Geometry check sheet. Reference: the model listing, model coordinates, mm. A direction names the side the tool comes from. Round coordinates to 2 decimals unless told otherwise and drop trailing zeros. Loops run counter-clockwise (first coordinate to the right, second up) from the corner with the lowest first, then second, coordinate; pieces in that order, holes last. Notation, with made-up numbers: (74.5, 55.25) - (123.5, 55.25) arc R26 ccw to (123.5, 72.25) - close; hole circle Ø2 at (16.25, -24.5). An arc over 180 degrees is marked (long way). Write item = value, one per line.
```python
from build123d import *

# Parameters (mm, degrees)
SKETCH_1_R               = 3.5
EXTRUDE_1_DEPTH          = 3
SKETCH_2_R               = 3
SKETCH_2_R_2             = 2.1
CUT_EXTRUDE_1_DEPTH      = 10
SKETCH_4_R               = 2.1
CUT_EXTRUDE_3_DEPTH      = 10
CHAMFER_1_SIZE           = 10
FILLET_1_R               = 3
SKETCH_5_R               = 2.1
CUT_EXTRUDE_4_DEPTH      = 10
SKETCH_3_R               = 1.6
CUT_EXTRUDE_5_DEPTH      = 10
EXTRUDE_2_DEPTH          = 6
CUT_EXTRUDE_6_DEPTH      = 182.747077005
CUT_EXTRUDE_6_DEPTH_BACK = 182.747077005
SKETCH_6_3_R             = 6.025
FILLET_2_R               = 6
SKETCH_7_R               = 2.1
EXTRUDE_3_DEPTH          = 6
FILLET_3_R               = 3


with BuildPart() as part:
    # 草图1 → 凸台-拉伸1 (new, symmetric)
    with BuildSketch(Plane(origin=(0, 0, 0), x_dir=(0, 0, -1), z_dir=(1, 0, 0))):
        with BuildLine():
            Line((-60, -42.021540511), (0, -70))
            Line((0, -70), (12, -70))
            Line((12, -70), (12, 30))
            Line((12, 30), (-75.715728753, 30))
            Line((-75.715728753, 30), (-125.857864376, 80.142135624))
            ThreePointArc((-125.857864376, 80.142135624), (-154.142135624, 80.142135624), (-154.142135624, 51.857864376))
            Line((-154.142135624, 51.857864376), (-92.284271247, -10))
            Line((-92.284271247, -10), (-60, -10))
            Line((-60, -10), (-60, -42.021540511))
        make_face()
        Circle(SKETCH_1_R, mode=Mode.SUBTRACT)
    extrude(amount=EXTRUDE_1_DEPTH, both=True)

    # 草图2 → 切除-拉伸1 (cut)
    with BuildSketch(Plane(origin=(3, 0, 0), x_dir=(0, 0, -1), z_dir=(1, 0, 0))):
        with Locations((-140, 66)):
            Circle(SKETCH_2_R)
        with Locations((-140, 82)):
            Circle(SKETCH_2_R_2)
        with Locations((-126.143593539, 74)):
            Circle(SKETCH_2_R_2)
        with Locations((-126.143593539, 58)):
            Circle(SKETCH_2_R_2)
        with Locations((-140, 50)):
            Circle(SKETCH_2_R_2)
        with Locations((-153.856406461, 58)):
            Circle(SKETCH_2_R_2)
        with Locations((-153.856406461, 74)):
            Circle(SKETCH_2_R_2)
    extrude(amount=-CUT_EXTRUDE_1_DEPTH, mode=Mode.SUBTRACT)

    # 草图4 → 切除-拉伸3 (cut)
    with BuildSketch(Plane(origin=(3, 0, 0), x_dir=(0, 0, -1), z_dir=(1, 0, 0))):
        with Locations((-55, -15)):
            Circle(SKETCH_4_R)
        with Locations((-55, -35)):
            Circle(SKETCH_4_R)
        with Locations((7, -65)):
            Circle(SKETCH_4_R)
        with Locations((7, -45)):
            Circle(SKETCH_4_R)
        with Locations((-8, -60.75264914)):
            Circle(SKETCH_4_R)
        with Locations((-26.126155741, -52.300283905)):
            Circle(SKETCH_4_R)
        with Locations((-44.252311481, -43.84791867)):
            Circle(SKETCH_4_R)
    extrude(amount=-CUT_EXTRUDE_3_DEPTH, mode=Mode.SUBTRACT)

    # 倒角1
    chamfer_1_edges = [part.edges().sort_by_distance(p)[0] for p in [
        (0, -10, 60),
    ]]
    chamfer(chamfer_1_edges, length=CHAMFER_1_SIZE)

    # 圆角1
    fillet_1_edges = [part.edges().sort_by_distance(p)[0] for p in [
        (0, -20, 60),
        (0, -10, 70),
        (0, 30, -12),
        (0, -70, -12),
        (0, -70, 0),
        (0, -42.021540511, 60),
        (0, -10, 92.284271247),
        (0, 30, 75.715728753),
    ]]
    fillet(fillet_1_edges, radius=FILLET_1_R)

    # 草图5 → 切除-拉伸4 (cut)
    with BuildSketch(Plane(origin=(3, 0, 0), x_dir=(0, 0, -1), z_dir=(1, 0, 0))):
        with Locations((-110, 57.213203436)):
            Circle(SKETCH_5_R)
        with Locations((-88.786796564, 36)):
            Circle(SKETCH_5_R)
        with Locations((-109.946763354, 14.785654888)):
            Circle(SKETCH_5_R)
        with Locations((-131.214342006, 35.94434337)):
            Circle(SKETCH_5_R)
        with Locations((-58, 25)):
            Circle(SKETCH_5_R)
        with Locations((-28, 25)):
            Circle(SKETCH_5_R)
    extrude(amount=-CUT_EXTRUDE_4_DEPTH, mode=Mode.SUBTRACT)

    # 草图3 → 切除-拉伸5 (cut)
    with BuildSketch(Plane(origin=(3, 0, 0), x_dir=(0, 0, -1), z_dir=(1, 0, 0))):
        with Locations((0, 8)):
            Circle(SKETCH_3_R)
        with Locations((6.92820323, 4)):
            Circle(SKETCH_3_R)
        with Locations((6.92820323, -4)):
            Circle(SKETCH_3_R)
        with Locations((0, -8)):
            Circle(SKETCH_3_R)
        with Locations((-6.92820323, -4)):
            Circle(SKETCH_3_R)
        with Locations((-6.92820323, 4)):
            Circle(SKETCH_3_R)
    extrude(amount=-CUT_EXTRUDE_5_DEPTH, mode=Mode.SUBTRACT)

    # 草图6 → 凸台-拉伸2 (add)
    with BuildSketch(Plane(origin=(3, 0, 0), x_dir=(0, 0, -1), z_dir=(1, 0, 0))):
        with BuildLine():
            ThreePointArc((-51.06307787, -50.273817383), (-46.226182617, -63.56307787), (-32.93692213, -58.726182617))
            ThreePointArc((-32.93692213, -58.726182617), (-32.302787653, -56.942145102), (-32.016290131, -55.070558726))
            Line((-32.016290131, -55.070558726), (-36.127383127, -53.153524579))
            ThreePointArc((-36.127383127, -53.153524579), (-36.013216988, -53.822464636), (-35.975, -54.5))
            ThreePointArc((-35.975, -54.5), (-45.144179406, -59.639529245), (-44.743385348, -49.13581676))
            Line((-44.743385348, -49.13581676), (-48.854478344, -47.218782613))
            ThreePointArc((-48.854478344, -47.218782613), (-50.10403963, -48.64128498), (-51.06307787, -50.273817383))
        make_face()
        with BuildLine():
            Line((-49.498462108, -46.918488052), (-51.06307787, -50.273817383))
            ThreePointArc((-51.06307787, -50.273817383), (-50.10403963, -48.64128498), (-48.854478344, -47.218782613))
            Line((-48.854478344, -47.218782613), (-49.498462108, -46.918488052))
        make_face()
        with BuildLine():
            ThreePointArc((-32.016290131, -55.070558726), (-32.302787653, -56.942145102), (-32.93692213, -58.726182617))
            Line((-32.93692213, -58.726182617), (-31.372306367, -55.370853287))
            Line((-31.372306367, -55.370853287), (-32.016290131, -55.070558726))
        make_face()
    extrude(amount=-EXTRUDE_2_DEPTH)

    # 草图6<3> → 切除-拉伸6 (cut, two sides: drawn at the far end of the back side and taken through both)
    with BuildSketch(Plane(origin=(3, 0, 0), x_dir=(0, 0, -1), z_dir=(1, 0, 0)).offset(-CUT_EXTRUDE_6_DEPTH_BACK)):
        with Locations((-42, -54.5)):
            Circle(SKETCH_6_3_R)
    extrude(amount=CUT_EXTRUDE_6_DEPTH + CUT_EXTRUDE_6_DEPTH_BACK, mode=Mode.SUBTRACT)

    # 圆角2
    fillet_2_edges = [part.edges().sort_by_distance(p)[0] for p in [
        (0, -46.918488052, 49.498462108),
        (0, -55.370853287, 31.372306367),
    ]]
    fillet(fillet_2_edges, radius=FILLET_2_R)

    # 草图7 → 凸台-拉伸3 (add)
    # profile 1 of 2: a face of its own
    with BuildSketch(Plane(origin=(3, 0, 0), x_dir=(0, 0, -1), z_dir=(1, 0, 0))):
        with BuildLine():
            Line((-61.377870017, 57.235829935), (-132.83107829, 84.671008583))
            ThreePointArc((-132.83107829, 84.671008583), (-129.106517373, 82.772955502), (-125.857864376, 80.142135624))
            Line((-125.857864376, 80.142135624), (-111.475100576, 65.759371824))
            Line((-111.475100576, 65.759371824), (-64.962330872, 47.900325644))
            Line((-64.962330872, 47.900325644), (-63.922837224, 50.607621888))
            ThreePointArc((-63.922837224, 50.607621888), (-65.130556346, 53.320814569), (-62.417363665, 54.528533691))
            Line((-62.417363665, 54.528533691), (-61.377870017, 57.235829935))
        make_face()
        with Locations((-81.841109028, 59.736999499)):
            Circle(SKETCH_7_R, mode=Mode.SUBTRACT)
    # profile 2 of 2: a face of its own
    with BuildSketch(Plane(origin=(3, 0, 0), x_dir=(0, 0, -1), z_dir=(1, 0, 0))):
        with BuildLine():
            Line((10.075338256, 29.800651288), (-61.377870017, 57.235829935))
            Line((-61.377870017, 57.235829935), (-62.417363665, 54.528533691))
            ThreePointArc((-62.417363665, 54.528533691), (-61.439385673, 53.757458461), (-61.070100444, 52.56807779))
            ThreePointArc((-61.070100444, 52.56807779), (-61.980719773, 50.837363019), (-63.922837224, 50.607621888))
            Line((-63.922837224, 50.607621888), (-64.962330872, 47.900325644))
            Line((-64.962330872, 47.900325644), (-18.342051383, 30))
            Line((-18.342051383, 30), (9, 30))
            ThreePointArc((9, 30), (9.546830018, 29.949741841), (10.075338256, 29.800651288))
        make_face()
        with Locations((-44.499091861, 45.39915608)):
            Circle(SKETCH_7_R, mode=Mode.SUBTRACT)
    extrude(amount=-EXTRUDE_3_DEPTH)

    # 圆角3
    fillet_3_edges = [part.edges().sort_by_distance(p)[0] for p in [
        (0, 65.759371824, 111.475100576),
        (0, 30, 18.342051383),
    ]]
    fillet(fillet_3_edges, radius=FILLET_3_R)


solid = part.part
```
(1) Gauge pin test, flat ends, axial feed: pin 1 (2.5 mm diameter, centred on y = 4, z = 6.93, fed in from +X); pin 2 (2 mm diameter, centred on x = -1.5, y = -16, fed in from +Z); pin 3 (3 mm diameter, centred on x = 1, z = 42.5, fed in from +Y); pin 4 (1 mm diameter, centred on x = 0.5, y = -5.5, fed in from +Z). Record the tip position at first contact, or that the pin passes through.
Answers follow:
pin_1 = through
pin_2 = 65
pin_3 = 50.56
pin_4 = 97.28
(2) Section check A-A (y = -35). Enter the section's corners in (x, z), then the cut area to 3 significant figures.
Answers follow:
outline = (-3, -12) - (3, -12) - (3, 52.9) - (-3, 52.9) - close; (-3, 57.1) - (3, 57.1) - (3, 60) - (-3, 60) - close
area = 407 mm²
(3) Section check C-C (x = -0.5). State how many separate pieces and enclosed holes the cut face has, then the cut area to 3 significant figures.
Answers follow:
separate_pieces = 1
enclosed_holes = 32
area = 12,200 mm²
(4) Section check B-B (y = 25). Enter the section's corners in (x, z).
Answers follow:
outline = (-3, -12) - (3, -12) - (3, 25.9) - (-3, 25.9) - close; (-3, 30.1) - (3, 30.1) - (3, 55.9) - (-3, 55.9) - close; (-3, 60.1) - (3, 60.1) - (3, 127.28) - (-3, 127.28) - close
(5) Mould release check, pull along Z, two halves, no side actions. Record for faces 1 (the cylindrical face through (0.042, 77.211, 156.562)), 2 (the cylindrical face through (0.042, 73.196, 151.917)), 3 (the flat face through (0, -70, -5)): pulls with the +Z half, pulls with the -Z half, needs draft (parallel to the pull), parting line crosses it, or undercut.
Answers follow:
face_1 = parting line crosses it
face_2 = undercut
face_3 = needs draft
(6) Scan lines: L1, parallel to Y at x = 0.5, z = 55; L2, parallel to Z at x = 1.75, y = 24.5; L3, parallel to Y at x = 2, z = 62. Record each from-to range of solid material in increasing order. Write a range as [from, to].
Answers follow:
L1 = [-44.35, -37.1], [-32.9, -17.1], [-12.9, 30], [44.08, 54.79]
L2 = [-12, 25.96], [30.04, 55.96], [60.04, 126.78]
L3 = [-18, 30], [46.76, 50.82], [54.31, 57.47]
(7) Set-up check for faces 4 (the flat face through (0, -21, -12)), 5 (the flat face through (0.042, 43.154, 88.869)), 6 (the flat face through (0, -10, 81)): record each of +Z, -Z, +X, -X, +Y, -Y from which the full face is reachable in a straight line by a thin tool's end or side.
Answers follow:
face_4 = -Z, +X, -X, +Y, -Y
face_5 = +X, -X
face_6 = +Z, +X, -X, -Y
